Can you work these out from the model? Positions are in its coordinate system, mm. Give positions to 0.01 mm unless a question says otherwise; leave off trailing zeros. Loops run counter-clockwise (first coordinate to the right, second up) from the corner with the lowest first, then second, coordinate; pieces in that order, holes last. Notation, with made-up numbers: (74, 9.5) - (102, 9.5) arc R22 ccw to (102, 16.5) - close; hole circle Ø9 at (83.5, -30.5). An arc over 180 degrees is marked (long way). Answer as a JSON object with one key per item and string values. Group by question number.
Item 1: Suppose I cut it at B-B on z = 651. Write out the boundary of the cut face in (x, y) (3 decimals).
Item 2: Will these pins go through, and if not, where does the flat tip stop? pin 1 (1 mm diameter, centred on x = 108.5, y = -2, fed in from -Z); pin 2 (1 mm diameter, centred on y = -1.5, z = 599.5, fed in from -X); pin 3 (2 mm diameter, centred on x = -77.5, z = 701, fed in from +Y); pin 4 (1.6 mm diameter, centred on y = -2, z = 737, fed in from +X).
Item 3: Thinking about a two-plate mould opening in X: for faces 1 (the flat face through (-2, -3.175, 669)), 2 (the cylindrical face through (81.734, -1.61, 635.912)), which applies, pulls with the +X half, pulls with the -X half, needs draft (parallel to the pull), parting line crosses it, or undercut?
Item 4: Please list where these lines run through material, in increasing order: L1, parallel to Z at x = -64, y = -2.05; L2, parallel to X at y = -2.95, z = 614 (3 decimals); L3, parallel to Z at x = 77, y = -1.05.
Item 5: Suppose I cut it at A-A on x = 14. Write out the boundary of the cut face in (y, z) (3 decimals), and give its area (3 significant figures).
from build123d import *

# Parameters (mm, degrees)
SKETCH48_W           = 219.999999786
SKETCH48_H           = 140
BOSS_EXTRUDE12_DEPTH = 3.175
SKETCH49_R           = 8
SKETCH49_W           = 20
SKETCH49_H           = 3.175
SKETCH49_W_2         = 3.175
SKETCH49_H_2         = 20
CUT_EXTRUDE24_DEPTH  = 3.175


with BuildPart() as part:
    # Sketch48 → Boss-Extrude12 (new body)
    with BuildSketch(Plane.XZ):
        with Locations((-4.307e-06, 668.101928689)):
            Rectangle(SKETCH48_W, SKETCH48_H)
    extrude(amount=BOSS_EXTRUDE12_DEPTH)

    # Sketch49 → Cut-Extrude24 (cut)
    with BuildSketch(Plane(origin=(0, -3.175, 0), x_dir=(-1, 0, 0), z_dir=(0, -1, 0))):
        with Locations((-79.999995586, -628.101928689)):
            Circle(SKETCH49_R)
        with Locations((60.0000042, -736.514428689)):
            Rectangle(SKETCH49_W, SKETCH49_H)
        Polygon((110.0000042, -738.101928689), (90.0000042, -738.101928689), (90.0000042, -734.926928689), (106.8250042, -734.926928689), (106.8250042, -718.101928689), (110.0000042, -718.101928689), align=None)
        with Locations((20.0000042, -736.514428689)):
            Rectangle(SKETCH49_W, SKETCH49_H)
        with Locations((-19.9999958, -736.514428689)):
            Rectangle(SKETCH49_W, SKETCH49_H)
        with Locations((-59.9999958, -736.514428689)):
            Rectangle(SKETCH49_W, SKETCH49_H)
        Polygon((-89.9999958, -738.101928689), (-89.9999958, -734.926928689), (-106.824995586, -734.926928689), (-106.824995586, -718.101928689), (-109.999995586, -718.101928689), (-109.9999958, -738.101928689), align=None)
        with Locations((60.0000042, -599.689428689)):
            Rectangle(SKETCH49_W, SKETCH49_H)
        Polygon((110.0000042, -598.101928689), (90.0000042, -598.101928689), (90.0000042, -601.276928689), (106.8250042, -601.276928689), (106.8250042, -618.101928689), (110.0000042, -618.101928689), align=None)
        with Locations((20.0000042, -599.689428689)):
            Rectangle(SKETCH49_W, SKETCH49_H)
        with Locations((-19.9999958, -599.689428689)):
            Rectangle(SKETCH49_W, SKETCH49_H)
        with Locations((-59.9999958, -599.689428689)):
            Rectangle(SKETCH49_W, SKETCH49_H)
        Polygon((-89.9999958, -598.101928689), (-89.9999958, -601.276928689), (-106.824995586, -601.276928689), (-106.824995586, -618.101928689), (-109.999995586, -618.101928689), (-109.9999958, -598.101928689), align=None)
        with Locations((108.4125042, -648.101928689)):
            Rectangle(SKETCH49_W_2, SKETCH49_H_2)
        with Locations((108.4125042, -688.101928689)):
            Rectangle(SKETCH49_W_2, SKETCH49_H_2)
        with Locations((-108.412495586, -648.101928689)):
            Rectangle(SKETCH49_W_2, SKETCH49_H_2)
        with Locations((-108.412495586, -688.101928689)):
            Rectangle(SKETCH49_W_2, SKETCH49_H_2)
    extrude(amount=-CUT_EXTRUDE24_DEPTH, mode=Mode.SUBTRACT)


solid = part.part
Worked out:
{
 "1": {"outline": "(-106.825, -3.175) - (106.825, -3.175) - (106.825, 0) - (-106.825, 0) - close"},
 "2": {"pin 1": "stops at z = 618.1", "pin 2": "stops at x = -90", "pin 3": "stops at y = 0", "pin 4": "stops at x = 90"},
 "3": {"face 1": "needs draft", "face 2": "undercut"},
 "4": {"L1": "z = 601.28 to 734.93", "L2": "x = -106.825 to 106.825", "L3": "z = 598.1 to 620.69, 635.52 to 738.1"},
 "5": {"outline": "(-3.175, 601.277) - (0, 601.277) - (0, 734.927) - (-3.175, 734.927) - close", "area": "424 mm2"}
}
